Autodesk Inventor part; units mm, degrees
ref_plane "YZ Plane" through (0, 0, 0) normal (1, 0, 0) x (0, 1, 0)
ref_plane "XZ Plane" through (0, 0, 0) normal (0, 1, 0) x (-1, 0, 0)
ref_plane "XY Plane" through (0, 0, 0) normal (0, 0, 1) x (1, 0, 0)
sketch "Block1" plane through (0, 0, 0) normal (0, 0, 1) x (1, 0, 0)
  circle A0 centre (-65.4812, 52.5391) radius 2.75 construction
  circle A1 centre (-65.4812, 52.5391) radius 5 construction
  line L0 (-55.4812, 62.5391) -> (-95.9812, 62.5391)
  line L1 (-95.9812, 62.5391) -> (-95.9812, 42.5391)
  arc A2 (-100.7311, 56.2391) -> (-100.7311, 58.8391) centre (-98.9812, 57.5391) ccw
  arc A3 (-100.7311, 46.2391) -> (-100.7311, 48.8391) centre (-98.9812, 47.5391) ccw
  line L2 (-95.9812, 42.5391) -> (-55.4812, 42.5391)
  arc A4 (-50.7312, 48.8391) -> (-50.7312, 46.2391) centre (-52.4812, 47.5391) ccw
  arc A5 (-50.7312, 58.8391) -> (-50.7312, 56.2391) centre (-52.4812, 57.5391) ccw
  line L3 (-55.4812, 62.5391) -> (-55.4812, 42.5391)
  point P0 (-74.5923, 52.5391)
sketch "open sketch to change param" plane through (0, 0, 0) normal (0, 0, 1) x (1, 0, 0)
  line L0 (0, 0) -> (450, 0)
  line L1 (450, 0) -> (450, 500)
  line L2 (0, 500) -> (0, 0)
  line L3 (225, 500) -> (225, 0) construction
  line L4 (0, 455) -> (5, 455)
  line L5 (5, 455) -> (5, 405)
  line L6 (5, 405) -> (0, 405)
  line L7 (0, 405) -> (0, 455)
  line L8 (450, 405) -> (450, 455)
  line L9 (100, 500) -> (100, 505)
  line L10 (100, 505) -> (50, 505)
  line L11 (50, 505) -> (50, 500)
  line L12 (50, 500) -> (0, 500)
  line L13 (200, 500) -> (200, 505)
  line L14 (200, 505) -> (150, 505)
  line L15 (150, 505) -> (150, 500)
  line L16 (300, 500) -> (300, 505)
  line L17 (300, 505) -> (250, 505)
  line L18 (250, 505) -> (250, 500)
  line L19 (400, 500) -> (400, 505)
  line L20 (400, 505) -> (350, 505)
  line L21 (350, 505) -> (350, 500)
  line L22 (150, 500) -> (100, 500)
  line L23 (250, 500) -> (200, 500)
  line L24 (450, 500) -> (400, 500)
  line L25 (350, 500) -> (300, 500)
  line L26 (5, 500) -> (5, 0)
  line L27 (445, 500) -> (445, 0)
  line L28 (0, 85) -> (5, 85)
  line L29 (0, 35) -> (5, 35)
  line L30 (450, 455) -> (445, 455)
  line L31 (445, 405) -> (450, 405)
  line L32 (450, 85) -> (445, 85)
  line L33 (450, 35) -> (445, 35)
  line L34 (0, 250) -> (445, 250)
  line L35 (100, 0) -> (100, -5)
  line L36 (100, -5) -> (50, -5)
  line L37 (50, -5) -> (50, 0)
  line L38 (200, 0) -> (200, -5)
  line L39 (200, -5) -> (150, -5)
  line L40 (150, -5) -> (150, 0)
  line L41 (300, 0) -> (300, -5)
  line L42 (300, -5) -> (250, -5)
  line L43 (250, -5) -> (250, 0)
  line L44 (400, 0) -> (400, -5)
  line L45 (400, -5) -> (350, -5)
  line L46 (350, -5) -> (350, 0)
  circle A0 centre (134.5, 132) radius 3.175
  line L47 (134.5, 132) -> (201.9264, 140.8134) construction
  line L48 (201.9264, 140.8134) -> (126.9265, 140.7316) construction
  line L49 (126.9265, 140.7316) -> (57.1208, 92.2325) construction
  line L50 (134.5, 132) -> (57.1208, 92.2325) construction
  line L51 (134.5, 132) -> (5, 132) construction
  circle A1 centre (57.1208, 92.2325) radius 3.175
  circle A2 centre (139.5, 145) radius 2.18
  circle A3 centre (129.5, 145) radius 2.18
  circle A4 centre (139.5, 98.5) radius 2.18
  circle A5 centre (129.5, 98.5) radius 2.18
  line L52 (201.9264, 140.8134) -> (-23.205, 247.8943) construction
  line L53 (133.9, 148) -> (133.9, 142)
  line L54 (133.9, 148) -> (135.1, 148)
  line L55 (135.1, 142) -> (135.1, 148)
  line L56 (133.9, 142) -> (135.1, 142)
  line L57 (135.1, 101.5) -> (133.9, 101.5)
  line L58 (133.9, 101.5) -> (133.9, 95.5)
  line L59 (133.9, 95.5) -> (135.1, 95.5)
  line L60 (135.1, 95.5) -> (135.1, 101.5)
  circle A6 centre (129.5, 145) radius 0.8
  circle A7 centre (139.5, 145) radius 0.8
  circle A8 centre (129.5, 98.5) radius 0.8
  circle A9 centre (139.5, 98.5) radius 0.8
  line L61 (0, 0) -> (0, 240)
  line L62 (0, 240) -> (-152.4, 240)
  line L63 (5, 0) -> (190, 0)
  line L64 (190, 0) -> (190, 190)
  line L65 (190, 190) -> (5, 190)
  line L66 (5, 190) -> (5, 0)
  circle A10 centre (134.5, 132) radius 2.75 construction
  circle A11 centre (134.5, 132) radius 5 construction
  line L67 (124.5, 142) -> (124.5, 101.5)
  line L68 (124.5, 101.5) -> (144.5, 101.5)
  arc A12 (130.8, 96.75) -> (128.2, 96.75) centre (129.5, 98.5) ccw
  arc A13 (140.8, 96.75) -> (138.2, 96.75) centre (139.5, 98.5) ccw
  line L69 (144.5, 101.5) -> (144.5, 142)
  arc A14 (138.2, 146.75) -> (140.8, 146.75) centre (139.5, 145) ccw
  arc A15 (128.2, 146.75) -> (130.8, 146.75) centre (129.5, 145) ccw
  line L70 (124.5, 142) -> (144.5, 142)
  point P0 (225, 240)
  point P1 (5, 480)
  point P2 (0, 455)
  point P3 (0, 405)
  point P4 (5, 405)
  point P5 (450, 35)
  point P6 (450, 85)
  point P7 (445, 85)
  point P8 (445, 405)
  point P9 (450, 405)
  point P10 (445, 35)
  point P11 (100, 0)
  point P12 (50, 0)
  point P13 (200, 0)
  point P14 (150, 0)
  point P15 (300, 0)
  point P16 (250, 0)
  point P17 (400, 0)
  point P18 (350, 0)
  point P19 (138.2, 146.75)
  point P20 (140.8, 146.75)
  point P21 (128.2, 146.75)
  point P22 (130.8, 146.75)
  point P23 (140.8, 96.75)
  point P24 (138.2, 96.75)
  point P25 (130.8, 96.75)
  point P26 (128.2, 96.75)
  point P27 (134.5, 142)
  point P28 (134.5, 142)
  point P29 (134.5, 101.5)
  point P30 (134.5, 101.5)
  point P31 (135.1, 101.5)
  point P32 (133.9, 101.5)
  dimension "d4" = 240
  dimension "d5" = 50
  dimension "d6" = 5
  dimension "d17" = 50
  dimension "d18" = 50
  dimension "d28" = 100
  dimension "d33" = 500
  dimension "d34" = 5
  dimension "d35" = 45
  dimension "d83" = 50
  dimension "d84" = 35
  dimension "d100" = 450
  dimension "d101" = 6.35
  dimension "d102" = 310.5
  dimension "d103" = 132
  dimension "d104" = -27.2
  dimension "d105" = 87
  dimension "d106" = 68
  dimension "d107" = 75
  dimension "d108" = 85
  dimension "d111" = 6.35
  dimension "d122" = 249.3
  dimension "d123" = 25.5
  dimension "d125" = 6
  dimension "d127" = 1.2
  dimension "d128" = 6
  dimension "d129" = 1.2
  dimension "d130" = 1.6
  dimension "d131" = 1.6
  dimension "d132" = 1.6
  dimension "d133" = 1.6
  dimension "d134" = 240
  dimension "d135" = 152.4
  dimension "d136" = 185
  dimension "d137" = 190
extrude "Extrusion1" add sketch "open sketch to change param" along normal blind 6.35 contours L26 L65 L64 L0 | L2 L28 L26 L29 | L0 L35 L36 L37 | L0 L38 L39 L40 | L26 L34 L27 L0 L64 L65 | L26 L5 L12 L11 L10 L9 L22 L15 L14 L13 L23 L18 L17 L16 L25 L21 L20 L19 L24 L27 L34 | L2 L4 L5 L6 | L0 L41 L42 L43 | L27 L30 L1 L31 | L32 L1 L33 L27 | L0 L44 L45 L46 | A2 | A3 | A4 | A5
sketch "Sketch2" plane through (0, 0, 6.35) normal (0, 0, 1) x (1, 0, 0)
  line L0 (0, 0) -> (0, -5)
  line L1 (0, -5) -> (190, -5)
  line L2 (190, -5) -> (190, 190)
  line L3 (190, 190) -> (0, 190)
  line L4 (0, 190) -> (0, -5)
  line L5 (0, 190) -> (0, 568.7197)
  line L6 (5, 405) -> (5, 85)
  line L7 (0, 568.7197) -> (531.5547, 568.7197)
  line L8 (531.5547, 568.7197) -> (531.5547, -5)
  line L9 (531.5547, -5) -> (190, -5)
  dimension "d138" = 5
  dimension "d139" = 190
  dimension "d140" = 195
extrude "Extrusion3" cut sketch "Sketch2" against normal blind 6.35 contours L5 L7 L8 L9 L2 L3
properties part number "Cut Pegboard Panel Skiba" material "Wood (Birch)"
CAD build for the part. Positions are in the model's coordinates, mm. A direction names the side the tool comes from. Round coordinates to 2 decimals unless told otherwise and drop trailing zeros. Order: outer loops, then holes, each group sorted by start corner. A loop starts at its lowest first (then second) coordinate and runs counter-clockwise, first axis right, second up. Notation, with made-up numbers: (68, 54) - (80, 54) arc R15 ccw to (80, 75) - close; hole circle Ø11 at (61.5, 44). An arc over 180 degrees is marked (long way). Return JSON: item names as keys, results as strings.
(1) Cut at C-C (x = 31). Give the cut face in (y, z).
Answer key:
{"outline": "(0, 0) - (190, 0) - (190, 6.35) - (0, 6.35) - close"}
(2) Tool access for faces 1 (the face through (125, 0, 3)), 2 (the face through (27, 0, 3)), 3 (the face through (129, 142, 3)), 4 (the face through (5, 138, 3)): list every direction of +Z, -Z, +X, -X, +Y, -Y with a clear straight run to the whole face (end or side of a thin tool).
Answer key:
{"face 1": "+Z, -Z, -Y", "face 2": "+Z, -Z, -X, -Y", "face 3": "+Z, -Z", "face 4": "+Z, -Z, -X, +Y"}
(3) Wall check: probe 1 along X at (y, z) = (98.5, 4.25); probe 2 along Y at (x, z) = (139.5, 2.5); probe 3 along X at (y, z) = (143, 2.5). Give the ranges that are in metal, low to high. Write a range as from..to.
Answer key:
{"probe 1": "x = 5..128.7, 130.3..133.9, 135.1..138.7, 140.3..190", "probe 2": "y = 0..97.7, 99.3..101.5, 142..144.2, 145.8..190", "probe 3": "x = 5..133.9, 135.1..190"}
(4) Pull direction X, two halves, no side cores. Call faces 5 (the face through (50, -3, 3)), 6 (the face through (140, 142, 3)), 7 (the face through (75, -5, 3)), 8 (the face through (135.1, 98, 3)): +X half, -X half, draft (parallel to the pull), parting line (faces both ways), or undercut.
Answer key:
{"face 5": "-X half", "face 6": "undercut", "face 7": "draft", "face 8": "undercut"}
(5) Cut at B-B (z = 2.5). State how many separate pieces and enclosed holes the cut face has, then the cut area to 3 significant figures.
Answer key:
{"separate pieces": "1", "enclosed holes": "6", "area": "35,000 mm^2"}
(6) Cut at A-A (y = 119.5). Give the cut face in (x, z).
Answer key:
{"outline": "(5, 0) - (124.5, 0) - (124.5, 6.35) - (5, 6.35) - close; (144.5, 0) - (190, 0) - (190, 6.35) - (144.5, 6.35) - close"}
(7) Pin check, flat tips, straight feed: pin 1 Ø3 at (y, z) = (120, 5.5) entering from -X; pin 2 Ø1.9 at (x, z) = (138.5, 3) entering from -Y; pin 3 Ø5 at (x, y) = (57.12, 92.23) entering from -Z; pin 4 Ø1.5 at (y, z) = (-3.5, 4) entering from -X. Stop position of each tip, or through.
Answer key:
{"pin 1": "stops at x = 5", "pin 2": "stops at y = 0", "pin 3": "passes through", "pin 4": "stops at x = 50"}
